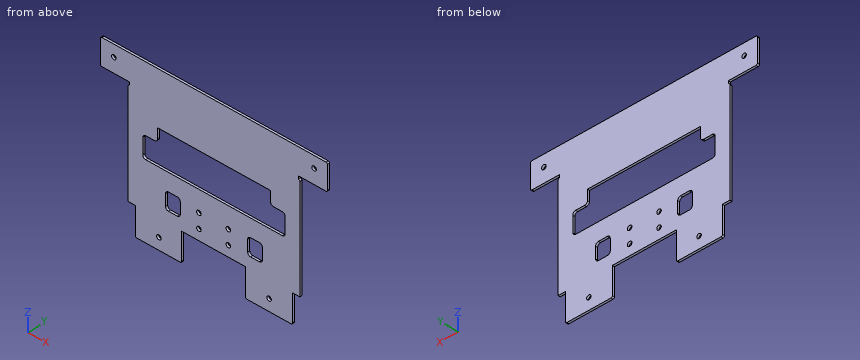
Autodesk Inventor part; units mm, degrees
ref_plane "YZ Plane" through (0, 0, 0) normal (1, 0, 0) x (0, 1, 0)
ref_plane "XZ Plane" through (0, 0, 0) normal (0, 1, 0) x (-1, 0, 0)
ref_plane "XY Plane" through (0, 0, 0) normal (0, 0, 1) x (1, 0, 0)
sketch "Sketch1" plane through (0, 0, 0) normal (0, 1, 0) x (-1, 0, 0)
  line L0 (-5, 55.3296) -> (112, 55.3296)
  line L1 (75.5, -0.4496) -> (107, -0.4496)
  line L2 (-5.1396, 93.9693) -> (-5.1396, 75.7793)
  line L3 (112.1396, 75.7793) -> (112.1396, 93.9693)
  line L4 (0, -0.4496) -> (32, -0.4496)
  arc A0 (30.54, 18.62) -> (28.54, 20.62) centre (28.54, 18.62) ccw
  line L5 (22.54, 20.62) -> (28.54, 20.62)
  arc A1 (28.54, 8.62) -> (30.54, 10.62) centre (28.54, 10.62) ccw
  line L6 (30.54, 18.62) -> (30.54, 10.62)
  arc A2 (22.54, 20.62) -> (20.54, 18.62) centre (22.54, 18.62) ccw
  line L7 (20.54, 10.62) -> (20.54, 18.62)
  arc A3 (20.54, 10.62) -> (22.54, 8.62) centre (22.54, 10.62) ccw
  line L8 (28.54, 8.62) -> (22.54, 8.62)
  arc A4 (78.46, 20.62) -> (76.46, 18.62) centre (78.46, 18.62) ccw
  line L9 (76.46, 10.62) -> (76.46, 18.62)
  arc A5 (86.46, 18.62) -> (84.46, 20.62) centre (84.46, 18.62) ccw
  line L10 (78.46, 20.62) -> (84.46, 20.62)
  arc A6 (76.46, 10.62) -> (78.46, 8.62) centre (78.46, 10.62) ccw
  line L11 (84.46, 8.62) -> (78.46, 8.62)
  arc A7 (84.46, 8.62) -> (86.46, 10.62) centre (84.46, 10.62) ccw
  line L12 (86.46, 18.62) -> (86.46, 10.62)
  arc A8 (7, 47.88) -> (5, 45.88) centre (7, 45.88) ccw
  line L13 (5, 34.88) -> (5, 45.88)
  arc A9 (13, 47.88) -> (15, 49.88) centre (13, 49.88) ccw
  line L14 (15, 49.88) -> (15, 56.9693)
  arc A10 (5, 34.88) -> (7, 32.88) centre (7, 34.88) ccw
  line L15 (100, 32.88) -> (7, 32.88)
  arc A11 (92, 49.88) -> (94, 47.88) centre (94, 49.88) ccw
  line L16 (92, 56.9693) -> (92, 49.88)
  arc A12 (102, 45.88) -> (100, 47.88) centre (100, 45.88) ccw
  line L17 (94, 47.88) -> (100, 47.88)
  arc A13 (100, 32.88) -> (102, 34.88) centre (100, 34.88) ccw
  line L18 (102, 45.88) -> (102, 34.88)
  line L19 (15, 56.9693) -> (92, 56.9693)
  line L20 (7, 47.88) -> (13, 47.88)
  circle A14 centre (91, -10.9943) radius 1.55
  circle A15 centre (16, -10.9943) radius 1.55
  circle A16 centre (121.6843, 85.8743) radius 1.55
  circle A17 centre (-14.6843, 85.8743) radius 1.55
  circle A18 centre (63.75, 8.19) radius 1.55
  circle A19 centre (63.75, 18.19) radius 1.55
  circle A20 centre (43.75, 8.19) radius 1.55
  circle A21 centre (43.75, 18.19) radius 1.55
  arc A22 (112, 72.7793) -> (111, 73.7793) centre (111, 72.7793) ccw
  arc A23 (-4, 73.7793) -> (-5, 72.7793) centre (-4, 72.7793) ccw
  line L21 (-3.94, 73.7793) -> (-4, 73.7793)
  arc A24 (-23.7793, 76.7793) -> (-22.7793, 75.7793) centre (-22.7793, 76.7793) ccw
  arc A25 (-22.7793, 93.9693) -> (-23.7793, 92.9693) centre (-22.7793, 92.9693) ccw
  line L22 (-22.7793, 93.9693) -> (129.7793, 93.9693)
  arc A26 (130.7793, 92.9693) -> (129.7793, 93.9693) centre (129.7793, 92.9693) ccw
  arc A27 (129.7793, 75.7793) -> (130.7793, 76.7793) centre (129.7793, 76.7793) ccw
  line L23 (129.7793, 75.7793) -> (110.94, 75.7793)
  arc A28 (31, -19.0893) -> (32, -18.0893) centre (31, -18.0893) ccw
  arc A29 (0, -18.0893) -> (1, -19.0893) centre (1, -18.0893) ccw
  arc A30 (106, -19.0893) -> (107, -18.0893) centre (106, -18.0893) ccw
  arc A31 (75.5, -18.0893) -> (76.5, -19.0893) centre (76.5, -18.0893) ccw
  line L24 (75.5, -18.0893) -> (75.5, 0.75)
  line L25 (106, -19.0893) -> (76.5, -19.0893)
  line L26 (107, 0.75) -> (107, -18.0893)
  line L27 (107, 0.75) -> (112, 0.75)
  line L28 (112, 72.7793) -> (112, 0.75)
  line L29 (31, -19.0893) -> (1, -19.0893)
  line L30 (0, -18.0893) -> (0, 0.75)
  line L31 (-5, 0.75) -> (0, 0.75)
  line L32 (32, 0.75) -> (32, -18.0893)
  line L33 (32, 0.75) -> (75.5, 0.75)
  line L34 (-5, 0.75) -> (-5, 72.7793)
  line L35 (130.7793, 92.9693) -> (130.7793, 76.7793)
  line L36 (-23.7793, 76.7793) -> (-23.7793, 92.9693)
  line L37 (-3.94, 75.7793) -> (-22.7793, 75.7793)
  line L38 (-3.94, 75.7793) -> (-3.94, 73.7793)
  line L39 (111, 73.7793) -> (110.94, 73.7793)
  line L40 (110.94, 73.7793) -> (110.94, 75.7793)
  line L41 (112.5893, 93.9693) -> (112.5893, 75.7793)
  line L42 (-5.5893, 75.7793) -> (-5.5893, 93.9693)
  line L43 (111.69, 75.7793) -> (111.69, 93.9693)
  line L44 (-4.69, 93.9693) -> (-4.69, 75.7793)
  line L45 (32, -0.8993) -> (0, -0.8993)
  line L46 (107, -0.8993) -> (75.5, -0.8993)
  line L47 (-5, 55.7793) -> (15, 55.7793)
  line L48 (92, 55.7793) -> (112, 55.7793)
  line L49 (0, 0) -> (32, 0)
  line L50 (75.5, 0) -> (107, 0)
  line L51 (15, 54.88) -> (-5, 54.88)
  line L52 (112, 54.88) -> (92, 54.88)
extrude "Extrusion1" add sketch "Sketch1" against normal blind 1.5 contours L34 L47 L14 L0 | L0 L14 L51 L34 | L51 L14 A9 L20 A8 L13 A10 L15 A13 L18 A12 L17 A11 L16 L52 L28 L27 L26 L50 L24 L33 L32 L49 L30 L31 L34 | L34 A23 L21 L38 L37 L44 L22 L43 L23 L40 L39 A22 L28 L48 L16 L19 L14 L47 | L16 L48 L28 L0 | L0 L28 L52 L16 | L49 L32 L4 L30 | L4 L32 L45 L30 | L45 L32 A28 L29 A29 L30 | L37 L2 L22 L44 | L26 L1 L24 L50 | L37 L42 L22 L2 | L26 L46 L24 L1 | L37 A24 L36 A25 L22 L42 | L22 L3 L23 L43 | L26 A30 L25 A31 L24 L46 | L22 L41 L23 L3 | L22 A26 L35 A27 L23 L41
properties part number "body_top_frame"
Verification items for the finished model (mm, model axes). Give positions to 0.01 mm unless a question says otherwise; leave off trailing zeros. Loops run counter-clockwise (first coordinate to the right, second up) from the corner with the lowest first, then second, coordinate; pieces in that order, holes last.
1. Section check A-A, the plane x = -81. Enter the section's corners in (y, z), then the cut area to 3 significant figures.
2. Section check C-C, the plane x = -63.75. Enter the section's corners in (y, z), then the cut area to 3 significant figures.
3. Section check D-D, the plane z = 14.5. Enter the section's corners in (x, y).
4. Thickness scan on line 1 (Z direction, x = -43.75, y = -0.9); line 2 (Z direction, x = -84, y = -0.3); line 3 (X direction, y = -0.5, z = 16). Record the ranges inside material, lowest first.
5. Section check B-B, the plane z = 42. Enter the section's corners in (x, y), then the cut area to 3 significant figures.
6. Go/stop test with flat-tipped pins: pin 1 Ø0.8 at (y, z) = (-1, 54.5) entering from -X; pin 2 Ø1.9 at (x, z) = (-121.68, 85.87) entering from +Y; pin 3 Ø0.8 at (x, y) = (-60, -0.5) entering from -Z; pin 4 Ø0.8 at (y, z) = (-1, -12) entering from -X. Record where each tip stops, or that it passes through.
Geometry says:
1. outline: (-1.5, -19.09) - (0, -19.09) - (0, 8.62) - (-1.5, 8.62) - close; (-1.5, 20.62) - (0, 20.62) - (0, 32.88) - (-1.5, 32.88) - close; (-1.5, 56.97) - (0, 56.97) - (0, 93.97) - (-1.5, 93.97) - close
1. area: 115 mm2
2. outline: (-1.5, 0.75) - (0, 0.75) - (0, 6.64) - (-1.5, 6.64) - close; (-1.5, 9.74) - (0, 9.74) - (0, 16.64) - (-1.5, 16.64) - close; (-1.5, 19.74) - (0, 19.74) - (0, 32.88) - (-1.5, 32.88) - close; (-1.5, 56.97) - (0, 56.97) - (0, 93.97) - (-1.5, 93.97) - close
2. area: 94.4 mm2
3. outline: (-112, -1.5) - (-86.46, -1.5) - (-86.46, 0) - (-112, 0) - close; (-76.46, -1.5) - (-30.54, -1.5) - (-30.54, 0) - (-76.46, 0) - close; (-20.54, -1.5) - (5, -1.5) - (5, 0) - (-20.54, 0) - close
4. line 1: z = 0.75 to 6.64, 9.74 to 16.64, 19.74 to 32.88, 56.97 to 93.97
4. line 2: z = -19.09 to 8.62, 20.62 to 32.88, 56.97 to 93.97
4. line 3: x = -112 to -86.46, -76.46 to -30.54, -20.54 to 5
5. outline: (-112, -1.5) - (-102, -1.5) - (-102, 0) - (-112, 0) - close; (-5, -1.5) - (5, -1.5) - (5, 0) - (-5, 0) - close
5. area: 30.0 mm2
6. pin 1: stops at x = -112
6. pin 2: passes through
6. pin 3: stops at z = 0.75
6. pin 4: stops at x = -107
